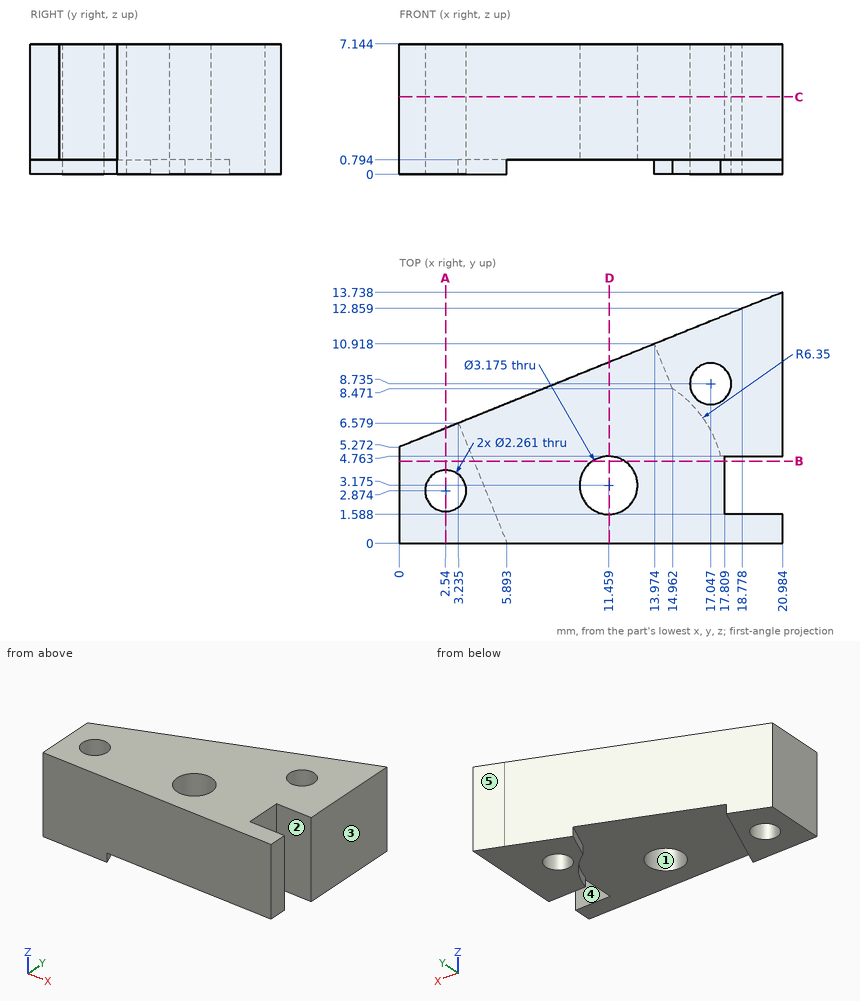
Study the drawing (mm; zero at the part's minimum x, y, z) and answer. A direction names the side the tool comes from. Round coordinates to 2 decimals unless told otherwise and drop trailing zeros. Write each loop counter-clockwise with the first axis right and the second up, starting at its lowest first coordinate (ties: lowest second). Pieces come first, ordered by that corner, then holes.
Q1. Straight lines are drawn through the part: line 1 (Z direction, x = 11, y = 9.25); line 2 (X direction, y = 9.5, z = 2.25) (1 decimal); line 3 (X direction, y = 2.25, z = 6). For each, find the intervals that lie inside material, in ascending order.
Values:
line 1: z = 0.79 to 7.14
line 2: x = 10.5 to 16.2, 17.9 to 21
line 3: x = 0 to 1.6, 3.48 to 10.17, 12.75 to 17.81
Q2. The mould has two halves that part along X. Classify the marked faces 1, 2 and 3: released by +X, released by -X, zero draft, split by the parting line, or undercut.
Values:
face 1: undercut
face 2: zero draft
face 3: released by +X
Q3. Find section C-C on z = 4.25. Determine the outline of the cut face in (x, y) (1 decimal).
Values:
outline: (0, 0) - (21, 0) - (21, 1.6) - (17.8, 1.6) - (17.8, 4.8) - (21, 4.8) - (21, 13.7) - (18.8, 12.9) - (0, 5.3) - close; hole circle Ø2.3 at (2.5, 2.9); hole circle Ø3.2 at (11.5, 3.2); hole circle Ø2.3 at (17, 8.7)
Q4. A tool of negligible diameter and unlimited length cuts with its end or side. For the marked faces 4 and 5, from which of +Z, -Z, +X, -X, +Y, -Y can it reach the whole face along a straight path? Write none if from no direction.
Values:
face 4: +Z, -Z, +X
face 5: +Z, -Z, -X, +Y
Q5. Flat-ended cylindrical pins translate along their axes: P1, Ø5.5, axis at x = 10, y = 3.5, coming from the -Z side; P2, Ø1.4, axis at x = 17.05, y = 8.74, coming from the -Z side; P3, Ø1, axis at y = 2.5, z = 4.5, coming from the +X side; P4, Ø1.6, axis at x = 19.5, z = 4, coming from the +Y side (1 decimal). Find the tip coordinate at first contact, or state that the pin passes through.
Values:
P1: stops at z = 0.79
P2: passes through
P3: stops at x = 17.81
P4: stops at y = 13.5
Q6. Find section B-B on y = 4.5. Determine the outline of the cut face in (x, z) (1 decimal), and give its area (3 significant figures).
Values:
outline: (0, 0) - (4.1, 0) - (4.1, 0.8) - (10.6, 0.8) - (10.6, 7.1) - (0, 7.1) - close; (12.3, 0.8) - (17.8, 0.8) - (17.8, 7.1) - (12.3, 7.1) - close
area: 105 mm2
Q7. Find section A-A on x = 2.54. Determine the outline of the cut face in (y, z) (1 decimal).
Values:
outline: (0, 0) - (1.7, 0) - (1.7, 7.1) - (0, 7.1) - close; (4, 0) - (6.3, 0) - (6.3, 7.1) - (4, 7.1) - close
Q8. Find section D-D on x = 11.5. Determine the outline of the cut face in (y, z).
Values:
outline: (0, 0.79) - (1.59, 0.79) - (1.59, 7.14) - (0, 7.14) - close; (4.76, 0.79) - (9.92, 0.79) - (9.92, 7.14) - (4.76, 7.14) - close
